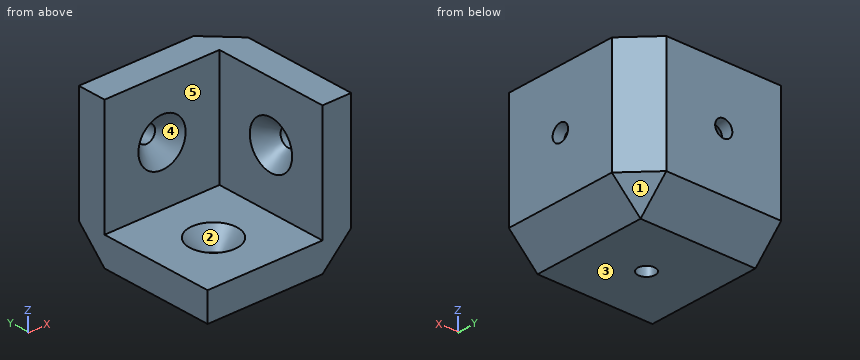
from build123d import *

# Parameters (mm, degrees)
F0_W                 = 25.4
F0_H                 = 25.4
F1_DEPTH             = 6.35
F2_W                 = 25.4
F2_H                 = 6.35
F3_DEPTH             = 6.35
F4_W                 = 25.4
F4_H                 = 6.35
F5_DEPTH             = 6.35
F9_D                 = 3.7973
F9_CSINK_D           = 10.4394
F9_CSINK_ANGLE       = 82
F9_ON_F6_D           = 3.7973
F9_ON_F6_CSINK_D     = 10.4394
F9_ON_F6_CSINK_ANGLE = 82
F9_ON_F8_D           = 3.7973
F9_ON_F8_CSINK_D     = 10.4394
F9_ON_F8_CSINK_ANGLE = 82
F10_SIZE             = 6.35


with BuildPart() as f1:
    # F0 (on Top) → F1 (new body)
    with BuildSketch(Plane.XY):
        Rectangle(F0_W, F0_H)
    extrude(amount=F1_DEPTH)

    # F2 (on face) → F3 (join)
    with BuildSketch(Plane.YZ.offset(12.7)):
        Polygon((12.7, 6.35), (12.7, 0), (19.05, 0), (19.05, 31.75), (-12.7, 31.75), (-12.7, 6.35), align=None)
        with Locations((0, 3.175)):
            Rectangle(F2_W, F2_H)
    extrude(amount=F3_DEPTH)

    # F4 (on face) → F5 (join)
    with BuildSketch(Plane(origin=(0, 12.7, 0), x_dir=(-1, 0, 0), z_dir=(0, 1, 0))):
        Polygon((-19.05, 0), (-12.7, 0), (-12.7, 6.35), (12.7, 6.35), (12.7, 31.75), (-19.05, 31.75), align=None)
        with Locations((0, 3.175)):
            Rectangle(F4_W, F4_H)
    extrude(amount=F5_DEPTH)

    # F9 (through all)
    with Locations(Plane(origin=(12.7, 0, 0), x_dir=(0, -1, 0), z_dir=(-1, 0, 0))):
        with Locations((0, 19.05)):
            CounterSinkHole(F9_D / 2, F9_CSINK_D / 2, counter_sink_angle=F9_CSINK_ANGLE)

    # F9 on F6 (through all)
    with Locations(Plane.XY.offset(6.35)):
        with Locations((0, 0)):
            CounterSinkHole(F9_ON_F6_D / 2, F9_ON_F6_CSINK_D / 2, counter_sink_angle=F9_ON_F6_CSINK_ANGLE)

    # F9 on F8 (through all)
    with Locations(Plane.XZ.offset(-12.7)):
        with Locations((0, 19.05)):
            CounterSinkHole(F9_ON_F8_D / 2, F9_ON_F8_CSINK_D / 2, counter_sink_angle=F9_ON_F8_CSINK_ANGLE)

    # F10
    f10_edges = [f1.edges().sort_by_distance(p)[0] for p in [
        (19.05, 19.05, 15.875),
        (19.05, 3.175, 0),
        (3.175, 19.05, 0),
    ]]
    chamfer(f10_edges, length=F10_SIZE)


solid = f1.part
The model under review builds one solid part; all positions refer to its coordinate system, in mm. Face numbers are marked on the shaded views. A direction names the side the tool comes from. Coordinates: 2 decimals unless noted, no trailing zeros. Write each loop counter-clockwise with the first axis right and the second up, starting at its lowest first coordinate (ties: lowest second). Pieces come first, ordered by that corner, then holes. Notation, with made-up numbers: M 28,-10 L 57,-10 A26 ccw 57,22 Z; hole C -29.5,83.25 d9. An arc over 180 degrees is marked long. Put each result on its own line as item: value.
1) For the marked faces 4 and 5, list the 3-axis set-ups (+Z, -Z, +X, -X, +Y, -Y) from which the entire face can be reached by the end or side of a thin tool; tool diameter is ignored.
Computed:
face 4: -Y
face 5: +Z, -X, -Y
2) Wall thickness on probe 1 along X at (y, z) = (8.5, 28.5); probe 2 along Z at (x, y) = (0, 17.25); probe 3 along X at (y, z) = (0, 1): over which ranges is each line inside the solid? List them lowest first. Write a range as [from, to].
Computed:
probe 1: x = [12.7, 19.05]
probe 2: z = [4.55, 17.15], [20.95, 31.75]
probe 3: x = [-12.7, -1.9], [1.9, 13.7]
3) Clearance check with flat-ended pins moving along their axes: pin 1 Ø4.5 at (y, z) = (0, 19.05) entering from +X; pin 2 Ø5 at (x, y) = (0, 0) entering from +Z; pin 3 Ø3 at (x, z) = (6, 27) entering from -Y; pin 4 Ø1.5 at (x, y) = (-4.5, 14) entering from -Z. State where each tip first meets the part, or that it passes through.
Computed:
pin 1: stops at x = 19.05
pin 2: stops at z = 3.22
pin 3: stops at y = 12.7
pin 4: stops at z = 0.55
4) Add section A-A on z = 19.05. Give the boundary of the cut face in (x, y).
Computed:
outline: M -12.7,12.7 L -5.22,12.7 L -1.9,16.52 L -1.9,19.05 L -12.7,19.05 Z; M 1.9,16.52 L 5.22,12.7 L 12.7,12.7 L 12.7,5.22 L 16.52,1.9 L 19.05,1.9 L 19.05,12.7 L 12.7,19.05 L 1.9,19.05 Z; M 12.7,-12.7 L 19.05,-12.7 L 19.05,-1.9 L 16.52,-1.9 L 12.7,-5.22 Z
5) Add section C-C on y = -10. Give the boundary of the cut face in (x, z).
Computed:
outline: M -12.7,0 L 12.7,0 L 19.05,6.35 L 19.05,31.75 L 12.7,31.75 L 12.7,6.35 L -12.7,6.35 Z
6) Draft analysis for pull direction X (two halves, no side actions). For the marked faces 1, 2 and 3, state which applies: released by +X, released by -X, zero draft, split by the parting line, or undercut.
Computed:
face 1: released by +X
face 2: undercut
face 3: zero draft
7) Add section B-B on x = 0. Give the boundary of the cut face in (y, z).
Computed:
outline: M -12.7,0 L -1.9,0 L -1.9,2.53 L -5.22,6.35 L -12.7,6.35 Z; M 1.9,0 L 12.7,0 L 19.05,6.35 L 19.05,17.15 L 16.52,17.15 L 12.7,13.83 L 12.7,6.35 L 5.22,6.35 L 1.9,2.53 Z; M 12.7,24.27 L 16.52,20.95 L 19.05,20.95 L 19.05,31.75 L 12.7,31.75 Z
